Design review of the part built by this model. Coordinates are the model's own, in mm. Face numbers are marked on the shaded views. Give positions to 0.01 mm unless a question says otherwise; leave off trailing zeros. Write each loop counter-clockwise with the first axis right and the second up, starting at its lowest first coordinate (ties: lowest second). Pieces come first, ordered by that corner, then holes. Notation, with made-up numbers: M 18.25,48.25 L 39.25,48.25 A16 ccw 39.25,75.25 Z; hole C 71,-20 d4. An arc over 180 degrees is marked long. Answer in a Markdown table with one row per item.
```python
from build123d import *

# Parameters (mm, degrees)
F0_R     = 43.75
F1_DEPTH = 37.5
F2_T     = -1
F3_R     = 7.5
F4_DEPTH = 25.4


with BuildPart() as f1:
    # F0 (on Top) → F1 (new body)
    with BuildSketch(Plane.XY):
        Circle(F0_R)
    extrude(amount=F1_DEPTH)

    # F2
    f2_openings = [f1.faces().sort_by_distance(p)[0] for p in [
        (0, 0, 37.5),
    ]]
    offset(amount=F2_T, openings=f2_openings)

    # F3 (on face) → F4 (cut)
    with BuildSketch(Plane(origin=(0, 0, 0), x_dir=(1, 0, 0), z_dir=(0, 0, -1))):
        Circle(F3_R)
    extrude(amount=-F4_DEPTH, mode=Mode.SUBTRACT)


solid = f1.part
```
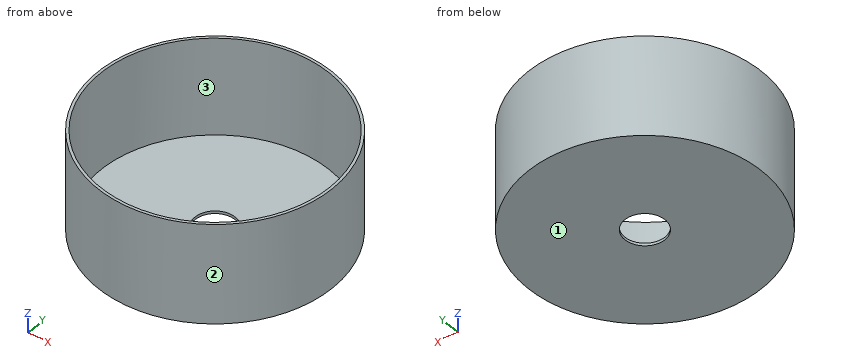
1) Add section D-D (y = -11). Write out the cut boundary in (x, z), and give its area (3 significant figures).
Geometry says:
| item | result |
|---|---|
| outline | M -42.34,0 L 42.34,0 L 42.34,37.5 L 41.31,37.5 L 41.31,1 L -41.31,1 L -41.31,37.5 L -42.34,37.5 Z |
| area | 160 mm^2 |
2) Add section A-A (y = 0). Write out the cut boundary in (x, z).
Geometry says:
| item | result |
|---|---|
| outline | M -43.75,0 L -7.5,0 L -7.5,1 L -42.75,1 L -42.75,37.5 L -43.75,37.5 Z; M 7.5,0 L 43.75,0 L 43.75,37.5 L 42.75,37.5 L 42.75,1 L 7.5,1 Z |
3) To check wall thickness, follow probe 1 along Y at (x, z) = (1, 25); probe 2 along Y at (x, z) = (0, 0.65); probe 3 along Z at (x, y) = (-28, -23.5). State the ranges of each line that lie inside material, in increasing order. Write a range as [from, to].
Geometry says:
| item | result |
|---|---|
| probe 1 | [-43.74, -42.74], [42.74, 43.74] |
| probe 2 | [-43.75, -7.5], [7.5, 43.75] |
| probe 3 | [0, 1] |
4) The part is to be moulded in two halves that separate along Y. For the marked faces 1, 2 and 3, say which applies: released by +Y, released by -Y, zero draft, split by the parting line, or undercut.
Geometry says:
| item | result |
|---|---|
| face 1 | zero draft |
| face 2 | split by the parting line |
| face 3 | undercut |
5) Insertion check: P1, Ø5, axis at x = -15.5, z = 28, coming from the +Y side; P2, Ø24, axis at x = 0, y = 0, coming from the +Z side; P3, Ø2, axis at y = 15, z = 10.5, coming from the -X side. Each pin has a flat end and moves straight along its axis. Give the tip position at first contact, or say it passes through.
Geometry says:
| item | result |
|---|---|
| P1 | y = 41.77 |
| P2 | z = 1 |
| P3 | x = -41.45 |
6) Add section C-C (z = 18). Write out the cut boundary in (x, y), and give its area (3 significant figures).
Geometry says:
| item | result |
|---|---|
| outline | C 0,0 d87.5; hole C 0,0 d85.5 |
| area | 272 mm^2 |
